Part model, mm, in its own coordinate system. A direction names the side the tool comes from. Round coordinates to 2 decimals unless told otherwise and drop trailing zeros. Loops run counter-clockwise (first coordinate to the right, second up) from the corner with the lowest first, then second, coordinate; pieces in that order, holes last. Notation, with made-up numbers: M 23.5,33 L 30.5,33 A26 ccw 30.5,55 Z; hole C 0.25,63.25 d4. An arc over 180 degrees is marked long. Put each result on its own line as item: value. Start each with the question number.
```python
from build123d import *

# Parameters (mm, degrees)
SKETCH1_R           = 2.0701
BOSS_EXTRUDE1_DEPTH = 2.286


with BuildPart() as part:
    # Sketch1 → Boss-Extrude1 (new body)
    with BuildSketch(Plane.XY.offset(2.286)):
        with BuildLine():
            Line((12.7, -54.991), (12.7, -6.35))
            ThreePointArc((12.7, -6.35), (14.559871939, -1.859871939), (19.05, 0))
            Line((19.05, 0), (42.291, 0))
            Line((42.291, 0), (44.45, 2.159))
            Line((44.45, 2.159), (44.45, 23.241))
            Line((44.45, 23.241), (42.291, 25.4))
            Line((42.291, 25.4), (-42.291, 25.4))
            Line((-42.291, 25.4), (-44.45, 23.241))
            Line((-44.45, 23.241), (-44.45, 2.159))
            Line((-44.45, 2.159), (-42.291, 0))
            Line((-42.291, 0), (-19.05, 0))
            ThreePointArc((-19.05, 0), (-14.559871939, -1.859871939), (-12.7, -6.35))
            Line((-12.7, -6.35), (-12.7, -54.991))
            Line((-12.7, -54.991), (-10.541, -57.15))
            Line((-10.541, -57.15), (10.541, -57.15))
            Line((10.541, -57.15), (12.7, -54.991))
        make_face()
        with Locations((0, -38.1)):
            Circle(SKETCH1_R, mode=Mode.SUBTRACT)
        with Locations((0, -12.7)):
            Circle(SKETCH1_R, mode=Mode.SUBTRACT)
        with Locations((38.1, 12.7)):
            Circle(SKETCH1_R, mode=Mode.SUBTRACT)
        with Locations((12.7, 12.7)):
            Circle(SKETCH1_R, mode=Mode.SUBTRACT)
        with Locations((-12.7, 12.7)):
            Circle(SKETCH1_R, mode=Mode.SUBTRACT)
        with Locations((-38.1, 12.7)):
            Circle(SKETCH1_R, mode=Mode.SUBTRACT)
        with Locations((-25.4, 12.7)):
            Circle(SKETCH1_R, mode=Mode.SUBTRACT)
        with Locations((0, 12.7)):
            Circle(SKETCH1_R, mode=Mode.SUBTRACT)
        with Locations((25.4, 12.7)):
            Circle(SKETCH1_R, mode=Mode.SUBTRACT)
        Circle(SKETCH1_R, mode=Mode.SUBTRACT)
        with Locations((0, -25.4)):
            Circle(SKETCH1_R, mode=Mode.SUBTRACT)
        with Locations((0, -50.8)):
            Circle(SKETCH1_R, mode=Mode.SUBTRACT)
    extrude(amount=-BOSS_EXTRUDE1_DEPTH)


solid = part.part
```
1. Cut at A-A, the plane x = 25.4. Give the cut face in (y, z).
2. Wall check: L1, parallel to X at y = -13, z = 1.7; L2, parallel to Y at x = 38, z = 0.35; L3, parallel to Y at x = 36.5, z = 1.85. Give the ranges that are in metal, low to high.
3. Cut at B-B, the plane y = 12.7. Give the number of separate pieces and of enclosed holes in the cut face, and give its area (3 significant figures).
4. Cut at C-C, the plane x = 0. Give the cut face in (y, z).
5. Which spindle directions (+Z, -Z, +X, -X, +Y, -Y) get a long thin tool onto all of the face, cutting with end or side? Do faces 4 (the cylindrical face through (12.431, 14.752, 1.159)), 5 (the flat face through (-31, 0, 1)). Say none if no direction does.
6. Mould opens along Y. For faces 1 (the flat face through (-12.7, -30, 1)), 2 (the flat face through (-43.355, 24.336, 1.159)), 3 (the cylindrical face through (26.513, 14.446, 1.159)) say: released by +Y, released by -Y, zero draft, split by the parting line, or undercut.
7. Drop flat-ended pins along their axis: pin 1 (6.5 mm diameter, centred on x = 0, y = -12.7, fed in from -Z); pin 2 (2.5 mm diameter, centred on x = 0, y = -50.8, fed in from +Z); pin 3 (1.1 mm diameter, centred on x = 33, z = 1.5, fed in from -Y); pin 4 (1.1 mm diameter, centred on y = -31, z = 1.5, fed in from +X). Give the stop position or say it passes through.
Results list:
1. outline: M 0,0 L 10.63,0 L 10.63,2.29 L 0,2.29 Z; M 14.77,0 L 25.4,0 L 25.4,2.29 L 14.77,2.29 Z
2. L1: x = -12.7 to -2.05, 2.05 to 12.7
2. L2: y = 0 to 10.63, 14.77 to 25.4
2. L3: y = 0 to 11.39, 14.01 to 25.4
3. separate pieces: 8
3. enclosed holes: 0
3. area: 137 mm^2
4. outline: M -57.15,0 L -52.87,0 L -52.87,2.29 L -57.15,2.29 Z; M -48.73,0 L -40.17,0 L -40.17,2.29 L -48.73,2.29 Z; M -36.03,0 L -27.47,0 L -27.47,2.29 L -36.03,2.29 Z; M -23.33,0 L -14.77,0 L -14.77,2.29 L -23.33,2.29 Z; M -10.63,0 L -2.07,0 L -2.07,2.29 L -10.63,2.29 Z; M 2.07,0 L 10.63,0 L 10.63,2.29 L 2.07,2.29 Z; M 14.77,0 L 25.4,0 L 25.4,2.29 L 14.77,2.29 Z
5. face 4: +Z, -Z
5. face 5: +Z, -Z, -X, -Y
6. face 1: zero draft
6. face 2: released by +Y
6. face 3: undercut
7. pin 1: stops at z = 0
7. pin 2: passes through
7. pin 3: stops at y = 0
7. pin 4: stops at x = 12.7
